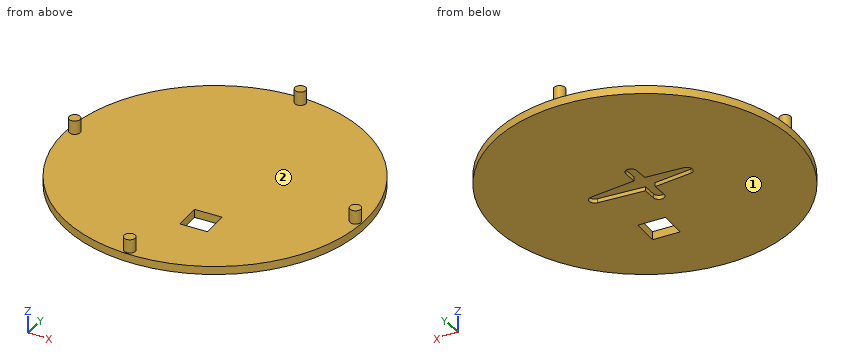
from build123d import *

# Parameters (mm, degrees)
SKETCH1_R           = 55
BOSS_EXTRUDE1_DEPTH = 3
SKETCH2_R           = 2
BOSS_EXTRUDE2_DEPTH = 5
CUT_EXTRUDE2_DEPTH  = 1.5
CUT_EXTRUDE3_DEPTH  = 23.5


with BuildPart() as part:
    # Sketch1 → Boss-Extrude1 (new body)
    with BuildSketch(Plane.XY):
        Circle(SKETCH1_R)
    extrude(amount=BOSS_EXTRUDE1_DEPTH)

    # Sketch2 → Boss-Extrude2 (add)
    with BuildSketch(Plane.XY.offset(3)):
        with Locations((0, 52.50213424)):
            Circle(SKETCH2_R)
        with Locations((52.50213424, 0)):
            Circle(SKETCH2_R)
        with Locations((0, -52.50213424)):
            Circle(SKETCH2_R)
        with Locations((-52.50213424, 0)):
            Circle(SKETCH2_R)
    extrude(amount=BOSS_EXTRUDE2_DEPTH)

    # Sketch5 → Cut-Extrude2 (cut)
    with BuildSketch(Plane(origin=(0, 0, 0), x_dir=(-1, 0, 0), z_dir=(0, 0, -1))):
        with BuildLine():
            Line((-2, 3.425408406), (-2, 8.425408406))
            ThreePointArc((-2, 8.425408406), (0, 10.425408406), (2, 8.425408406))
            Line((2, 8.425408406), (2, 3.425408406))
            Line((2, 3.425408406), (15.926066161, 1.98850852))
            ThreePointArc((15.926066161, 1.98850852), (17.719893525, 0.015831878), (15.957535976, -1.985009349))
            Line((15.957535976, -1.985009349), (2, -3.074591594))
            Line((2, -3.074591594), (2, -8.574591594))
            ThreePointArc((2, -8.574591594), (0, -10.574591594), (-2, -8.574591594))
            Line((-2, -8.574591594), (-2, -3.574591594))
            Line((-2, -3.574591594), (-18.913070191, -1.874440835))
            ThreePointArc((-18.913070191, -1.874440835), (-20.71285333, 0.115332129), (-18.913070191, 2.105105093))
            Line((-18.913070191, 2.105105093), (-2, 3.425408406))
        make_face()
    extrude(amount=-CUT_EXTRUDE2_DEPTH, mode=Mode.SUBTRACT)

    # Sketch7 → Cut-Extrude3 (cut)
    with BuildSketch(Plane(origin=(0, 0, 0), x_dir=(-1, 0, 0), z_dir=(0, 0, -1))):
        Polygon((-14.927590982, -20.209975768), (-15.441616431, -30.196755922), (-5.454836278, -30.710781371), (-4.940810829, -20.724001217), align=None)
    extrude(amount=-CUT_EXTRUDE3_DEPTH, mode=Mode.SUBTRACT)


solid = part.part
Part model, mm, in its own coordinate system. Face numbers are marked on the shaded views. A direction names the side the tool comes from. Round coordinates to 2 decimals unless told otherwise and drop trailing zeros. Loops run counter-clockwise (first coordinate to the right, second up) from the corner with the lowest first, then second, coordinate; pieces in that order, holes last. Notation, with made-up numbers: (34.5, 69.5) - (82.5, 69.5) arc R16 cw to (82.5, 91.5) - close; hole circle Ø6 at (-32, -1.5). An arc over 180 degrees is marked (long way). Answer as a JSON object with one key per item and string values.
Item 1: Band-saw the part on D-D on y = 0. List the corners of the cut face in (x, z), plus the area to 3 significant figures.
Output:
{"outline": "(-55, 0) - (-17.72, 0) - (-17.72, 1.5) - (20.71, 1.5) - (20.71, 0) - (55, 0) - (55, 3) - (54.5, 3) - (54.5, 8) - (50.5, 8) - (50.5, 3) - (-50.5, 3) - (-50.5, 8) - (-54.5, 8) - (-54.5, 3) - (-55, 3) - close", "area": "312 mm2"}
Item 2: Wall check: L1, parallel to Z at x = 36, y = -29; L2, parallel to X at y = -8.5, z = 0.5; L3, parallel to Y at x = 35, z = 1.25. Give the ranges that are in metal, low to high.
Output:
{"L1": "0 to 3", "L2": "-54.34 to -2, 2 to 54.34", "L3": "-42.43 to 42.43"}
Item 3: Band-saw the part on A-A on y = -28. List the corners of the cut face in (x, z), plus the area to 3 significant figures.
Output:
{"outline": "(-47.34, 0) - (5.32, 0) - (5.32, 3) - (-47.34, 3) - close; (15.33, 0) - (47.34, 0) - (47.34, 3) - (15.33, 3) - close", "area": "254 mm2"}
Item 4: Pin check, flat tips, straight feed: pin 1 (23 mm diameter, centred on x = 1, y = 4, fed in from -Z); pin 2 (1.6 mm diameter, centred on y = -5.5, z = 1, fed in from +X); pin 3 (1.5 mm diameter, centred on x = -37, y = 17, fed in from +Z); pin 4 (1.2 mm diameter, centred on y = -5, z = 0.5, fed in from -X). Stop position of each tip, or through.
Output:
{"pin 1": "z = 0", "pin 2": "x = 54.8", "pin 3": "z = 3", "pin 4": "x = -54.82"}
Item 5: Tool access for the marked faces 1 and 2: list every direction of +Z, -Z, +X, -X, +Y, -Y with a clear straight run to the whole face (end or side of a thin tool).
Output:
{"face 1": "-Z, +X, -X, +Y, -Y", "face 2": "+Z"}
Item 6: Band-saw the part on C-C on z = 6.75. List the corners of the cut face in (x, y).
Output:
{"outline": "circle Ø4 at (-52.5, 0); circle Ø4 at (0, -52.5); circle Ø4 at (0, 52.5); circle Ø4 at (52.5, 0)"}
Item 7: Band-saw the part on B-B on x = 0. List the corners of the cut face in (y, z), plus the area to 4 significant figures.
Output:
{"outline": "(-55, 0) - (-10.57, 0) - (-10.57, 1.5) - (10.43, 1.5) - (10.43, 0) - (55, 0) - (55, 3) - (54.5, 3) - (54.5, 8) - (50.5, 8) - (50.5, 3) - (-50.5, 3) - (-50.5, 8) - (-54.5, 8) - (-54.5, 3) - (-55, 3) - close", "area": "338.5 mm2"}
